from build123d import *

# Parameters (mm, degrees)
F0_R     = 3
F1_DEPTH = 3
F2_START = -14.5
F2_DEPTH = 1.5
F3_START = 16
F3_DEPTH = 2
F6_DEPTH = 18.001
F7_DEPTH = 1.175
F8_DEPTH = 1.175
F9_DEPTH = 100


with BuildPart() as f1:
    # F0 (on Top) → F1 (new body)
    with BuildSketch(Plane.XY):
        with BuildLine():
            ThreePointArc((5.2, -10.2571925984), (9.799234664, -6.0187207943), (11.5, 0))
            ThreePointArc((11.5, 0), (-8.5454666344, 7.6957780633), (1.2, -11.4372199419))
            Line((1.2, -11.4372199419), (1.2, -4.1398492453))
            ThreePointArc((1.2, -4.1398492453), (3.2, -2.1398492453), (5.2, -4.1398492453))
            Line((5.2, -4.1398492453), (5.2, -10.2571925984))
        make_face()
        Circle(F0_R, mode=Mode.SUBTRACT)
        Circle(F0_R)
    extrude(amount=F1_DEPTH)

    # F0 (on Top) → F6 (cut, through all)
    with BuildSketch(Plane.XY):
        with BuildLine():
            Line((1.2, -4.1398492453), (1.2, -11.4372199419))
            ThreePointArc((1.2, -11.4372199419), (3.253938557, -11.0300445995), (5.2, -10.2571925984))
            Line((5.2, -10.2571925984), (5.2, -4.1398492453))
            ThreePointArc((5.2, -4.1398492453), (3.2, -2.1398492453), (1.2, -4.1398492453))
        make_face()
        with BuildLine():
            ThreePointArc((5.2, -10.2571925984), (3.253938557, -11.0300445995), (1.2, -11.4372199419))
            Line((1.2, -11.4372199419), (1.2, -11.9398492453))
            ThreePointArc((1.2, -11.9398492453), (3.2490662236, -11.5517777279), (5.2, -10.8148046677))
            Line((5.2, -10.8148046677), (5.2, -10.2571925984))
        make_face()
    extrude(amount=F6_DEPTH, mode=Mode.SUBTRACT)



with BuildPart() as f2:
    # F1_face (on face) → F2 (new body)
    with BuildSketch(Plane(origin=(-0.2778637097, 0.5964787123, 0), x_dir=(1, 0, 0), z_dir=(0, 0, -1)).offset(F2_START)):
        with BuildLine():
            ThreePointArc((1.4778637097, 12.0336986542), (-2.9760748473, -10.4335658873), (5.4778637097, 10.8536713106))
            Line((5.4778637097, 10.8536713106), (5.4778637097, 4.7363279575))
            ThreePointArc((5.4778637097, 4.7363279575), (3.4778637097, 2.7363279575), (1.4778637097, 4.7363279575))
            Line((1.4778637097, 4.7363279575), (1.4778637097, 12.0336986542))
        make_face()
    extrude(amount=-F2_DEPTH)


with BuildPart() as f3:
    # F0 (on Top) → F3 (new body)
    with BuildSketch(Plane.XY.offset(F3_START)):
        with BuildLine():
            ThreePointArc((5.2, -10.2571925984), (9.799234664, -6.0187207943), (11.5, 0))
            ThreePointArc((11.5, 0), (-8.5454666344, 7.6957780633), (1.2, -11.4372199419))
            Line((1.2, -11.4372199419), (1.2, -4.1398492453))
            ThreePointArc((1.2, -4.1398492453), (3.2, -2.1398492453), (5.2, -4.1398492453))
            Line((5.2, -4.1398492453), (5.2, -10.2571925984))
        make_face()
        Circle(F0_R, mode=Mode.SUBTRACT)
        with BuildLine():
            ThreePointArc((1.2, -11.4372199419), (-8.5454666344, 7.6957780633), (11.5, 0))
            ThreePointArc((11.5, 0), (9.799234664, -6.0187207943), (5.2, -10.2571925984))
            Line((5.2, -10.2571925984), (5.2, -10.8148046677))
            ThreePointArc((5.2, -10.8148046677), (10.1587400794, -6.3874877691), (12, 0))
            ThreePointArc((12, 0), (-8.8994381845, 8.049844719), (1.2, -11.9398492453))
            Line((1.2, -11.9398492453), (1.2, -11.4372199419))
        make_face()
        Circle(F0_R)
    extrude(amount=F3_DEPTH)


with BuildPart() as f7:
    # F4 (on Front) → F7 (new body, symmetric)
    with BuildSketch(Plane.XZ):
        Polygon((-11.25, 30), (-11.25, 0), (0, 0), (11.25, 0), (11.25, 30), (7, 100), (0, 125), (-7, 100), align=None)
    extrude(amount=F7_DEPTH, both=True)


with BuildPart() as f8:
    # F5 (on Right) → F8 (new body, symmetric)
    with BuildSketch(Plane.YZ):
        Polygon((-11.25, 30), (-11.25, 0), (0, 0), (11.25, 0), (11.25, 30), (7, 100), (0, 125), (-7, 100), align=None)
    extrude(amount=F8_DEPTH, both=True)


with BuildPart() as f1_1:
    add(f1.part)

    add(f2.part)  # F9 merges F2

    add(f3.part)  # F9 merges F3

    add(f7.part)  # F9 merges F7

    add(f8.part)  # F9 merges F8
    # F0 (on Top) → F9 (join)
    with BuildSketch(Plane.XY):
        Circle(F0_R)
    extrude(amount=F9_DEPTH)


solid = f1_1.part
Can you work these out from the model? Positions are in its coordinate system, mm. A direction names the side the tool comes from. Coordinates: 2 decimals unless noted, no trailing zeros. Order: outer loops, then holes, each group sorted by start corner. A loop starts at its lowest first (then second) coordinate and runs counter-clockwise, first axis right, second up. Notation, with made-up numbers: (42.25, 10) -> (97.25, 10) arc R9 cw to (97.25, 23) -> close; hole circle Ø11 at (-22, -37). An arc over 180 degrees is marked (long way). Use one line per item in the form item = value.
Q1. Imagine slicing it at B-B, the plane y = -8.75. List the corners of the cut face in (x, z) for me (3 decimals), then the cut area to 3 significant figures.
From the geometry:
outline = (-8.212, 16) -> (-7.462, 16) -> (-7.462, 14.5) -> (-1.175, 14.5) -> (-1.175, 3) -> (-7.462, 3) -> (-7.462, 0) -> (1.2, 0) -> (1.2, 3) -> (1.175, 3) -> (1.175, 14.5) -> (1.2, 14.5) -> (1.2, 18) -> (1.175, 18) -> (1.175, 71.176) -> (-1.175, 71.176) -> (-1.175, 18) -> (-8.212, 18) -> close; (5.2, 0) -> (7.462, 0) -> (7.462, 3) -> (5.2, 3) -> close; (5.2, 14.5) -> (7.462, 14.5) -> (7.462, 16) -> (8.212, 16) -> (8.212, 18) -> (5.2, 18) -> close
area = 226 mm²
Q2. We'd pull the mould along X, two halves only. Please class faces 1 (the face through (-6, -1.175, 59)), 2 (the face through (-3.708, 10.886, 15.24)), 3 (the face through (1.2, -8, 16)), 4 (the face through (11.25, 0, 9)): released by +X, released by -X, zero draft, split by the parting line, or undercut.
From the geometry:
face_1 = zero draft
face_2 = split by the parting line
face_3 = undercut
face_4 = released by +X
Q3. Imagine slicing it at D-D, the plane z = 108. List the corners of the cut face in (x, y) for me (3 decimals).
From the geometry:
outline = (-4.76, -1.175) -> (-1.175, -1.175) -> (-1.175, -4.76) -> (1.175, -4.76) -> (1.175, -1.175) -> (4.76, -1.175) -> (4.76, 1.175) -> (1.175, 1.175) -> (1.175, 4.76) -> (-1.175, 4.76) -> (-1.175, 1.175) -> (-4.76, 1.175) -> close
Q4. Imagine slicing it at C-C, the plane y = 8.5. List the corners of the cut face in (x, z) for me (3 decimals), then the cut area to 3 significant figures.
From the geometry:
outline = (-8.471, 16) -> (-7.746, 16) -> (-7.746, 14.5) -> (-1.175, 14.5) -> (-1.175, 3) -> (-7.746, 3) -> (-7.746, 0) -> (7.746, 0) -> (7.746, 3) -> (1.175, 3) -> (1.175, 14.5) -> (7.746, 14.5) -> (7.746, 16) -> (8.471, 16) -> (8.471, 18) -> (1.175, 18) -> (1.175, 75.294) -> (-1.175, 75.294) -> (-1.175, 18) -> (-8.471, 18) -> close
area = 265 mm²
Q5. Which directions (+Z, -Z, +X, -X, +Y, -Y) give clear straight access to the entire face, cutting with the end or side of a thin tool? Please do faces 5 (the face through (-1.175, 6, 59)), 6 (the face through (1.175, 7, 9)), 7 (the face through (2.4, 2.4, 14.5)).
From the geometry:
face_5 = +Z, -X, +Y
face_6 = +X, +Y
face_7 = none
Q6. Will these pins go through, and if not, where does the flat tip stop? P1, Ø1, axis at x = 7.5, y = -4, coming from the -Z side; P2, Ø7, axis at y = -8, z = 9, coming from the -X side (3 decimals); P3, Ø9.5, axis at y = 6.5, z = 6.5, coming from the -X side; P4, Ø3, axis at x = 4, z = 35, coming from the +Y side.
From the geometry:
P1 = 0
P2 = -1.175
P3 = -11.02
P4 = 1.66
Q7. I need wall thicknesses on L1, parallel to Z at x = -5, y = 3.5; L2, parallel to X at y = -9.5, z = 22 (3 decimals); L3, parallel to Z at x = 3.75, y = 11. Which ranges of each line are inside material? Lowest first, please.
From the geometry:
L1 = 0 to 3, 14.5 to 18
L2 = -1.175 to 1.175
L3 = 16 to 18
Q8. Imagine slicing it at A-A, the plane z = 86. List the corners of the cut face in (x, y) for me (3 decimals), then the cut area to 3 significant figures.
From the geometry:
outline = (-7.85, -1.175) -> (-2.76, -1.175) arc R3 ccw to (-1.175, -2.76) -> (-1.175, -7.85) -> (1.175, -7.85) -> (1.175, -2.76) arc R3 ccw to (2.76, -1.175) -> (7.85, -1.175) -> (7.85, 1.175) -> (2.76, 1.175) arc R3 ccw to (1.175, 2.76) -> (1.175, 7.85) -> (-1.175, 7.85) -> (-1.175, 2.76) arc R3 ccw to (-2.76, 1.175) -> (-7.85, 1.175) -> close
area = 74.6 mm²
